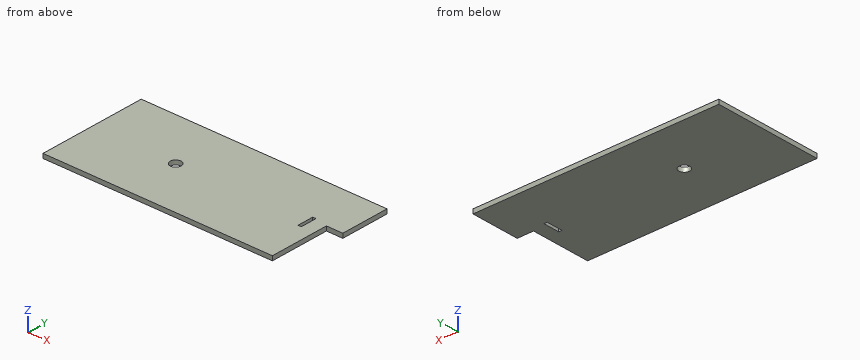
from build123d import *

# Parameters (mm, degrees)
SKETCH1_R           = 5
SKETCH1_W           = 3
SKETCH1_H           = 15
BOSS_EXTRUDE1_DEPTH = 4


with BuildPart() as part:
    # Sketch1 → Boss-Extrude1 (new body)
    with BuildSketch(Plane.XY):
        Polygon((60, 50), (75, 50), (75, 5), (60, 5), (60, -50), (-150, -50), (-150, 50), align=None)
        with Locations((-73.5, 0)):
            Circle(SKETCH1_R, mode=Mode.SUBTRACT)
        with Locations((46.5, 0.26206532)):
            Rectangle(SKETCH1_W, SKETCH1_H, mode=Mode.SUBTRACT)
    extrude(amount=BOSS_EXTRUDE1_DEPTH)


solid = part.part
Build history of the part. All positions in model axes, mm. Coordinates: 2 decimals unless noted, no trailing zeros. Order: outer loops, then holes, each group sorted by start corner. A loop starts at its lowest first (then second) coordinate and runs counter-clockwise, first axis right, second up. Notation, with made-up numbers: (53, 87) - (104, 87) arc R8 ccw to (104, 96) - close; hole circle Ø4 at (30.25, 31). An arc over 180 degrees is marked (long way). Write item = value, one per line. Start each with the question number.
1) Wall check: line 1 along Y through (x, z) = (-73.5, 0.8); line 2 along X through (y, z) = (-3.5, 3.45); line 3 along X through (y, z) = (-34, 1.85). Give the ranges that are in metal, low to high. Write a range as from..to.
2) Saw through at B-B on y = 0. Write the cut outline in (x, z), then the cut area to 3 significant figures.
3) Saw through at C-C on z = 0.7. Write the cut outline in (x, y), then the cut area to 3 significant figures.
4) Saw through at D-D on y = -26. Write the cut outline in (x, z).
5) Saw through at A-A on x = -73.5. Write the cut outline in (y, z).
6) Flat gauge pins, fed straight in: pin 1 Ø2 at (x, z) = (66.5, 2.5) entering from -Y; pin 2 Ø2 at (y, z) = (-23, 2) entering from +X. Where does each tip first touch, or does it go through?
From the geometry:
q1.line_1 = -50..-5, 5..50
q1.line_2 = -150..-77.07, -69.93..45, 48..60
q1.line_3 = -150..60
q2.outline = (-150, 0) - (-78.5, 0) - (-78.5, 4) - (-150, 4) - close; (-68.5, 0) - (45, 0) - (45, 4) - (-68.5, 4) - close; (48, 0) - (60, 0) - (60, 4) - (48, 4) - close
q2.area = 788 mm^2
q3.outline = (-150, -50) - (60, -50) - (60, 5) - (75, 5) - (75, 50) - (-150, 50) - close; hole circle Ø10 at (-73.5, 0); hole (45, -7.24) - (48, -7.24) - (48, 7.76) - (45, 7.76) - close
q3.area = 21,600 mm^2
q4.outline = (-150, 0) - (60, 0) - (60, 4) - (-150, 4) - close
q5.outline = (-50, 0) - (-5, 0) - (-5, 4) - (-50, 4) - close; (5, 0) - (50, 0) - (50, 4) - (5, 4) - close
q6.pin_1 = 5
q6.pin_2 = 60
